from build123d import *

# Parameters (mm, degrees)
F1_DEPTH = 76.2
F2_R     = 4.5085
F3_DEPTH = 92.761762
F4_R     = 6.35
F5_DEPTH = 118.672617


with BuildPart() as f1:
    # F0 (on Front) → F1 (new body)
    with BuildSketch(Plane.XZ):
        Polygon((-46.039158, 105.114406), (-96.838128, 105.437962), (-96.838128, -97.762038), (55.561872, -97.762038), (55.561872, -46.962038), (-46.039158, -46.962038), align=None)
    extrude(amount=F1_DEPTH)

    # F2 (on face) → F3 (cut)
    with BuildSketch(Plane.XY.offset(-46.962038)):
        with Locations((15.037069, -37.766326)):
            Circle(F2_R)
    extrude(amount=-F3_DEPTH, mode=Mode.SUBTRACT)

    # F4 (on face) → F5 (cut)
    with BuildSketch(Plane.YZ.offset(-46.039158)):
        with Locations((-38.88151, 66.329271)):
            Circle(F4_R)
    extrude(amount=-F5_DEPTH, mode=Mode.SUBTRACT)


solid = f1.part
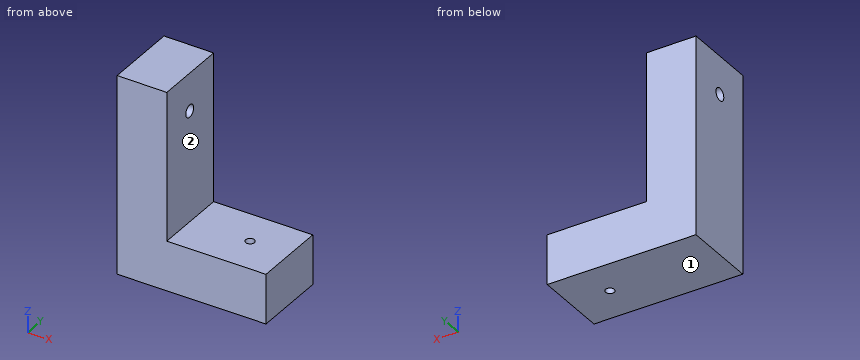
Work out the finished part from the listing and answer in its coordinate system (mm). Face numbers are marked on the shaded views. A direction names the side the tool comes from. Give positions to 0.01 mm unless a question says otherwise; leave off trailing zeros. Order: outer loops, then holes, each group sorted by start corner. A loop starts at its lowest first (then second) coordinate and runs counter-clockwise, first axis right, second up. Notation, with made-up numbers: M 58.5,-25 L 62.5,-25 A22 ccw 62.5,-7 Z; hole C -7,77.5 d10. An arc over 180 degrees is marked long. Return JSON: item names as keys, results as strings.
Q1. Find section B-B, the plane x = -12.5. Write down the section's boundary in (y, z).
Answer below:
{"outline": "M -76.2,-97.76 L 0,-97.76 L 0,-46.96 L -76.2,-46.96 Z"}
Q2. Which of the six approach directions +Z, -Z, +X, -X, +Y, -Y give full straight-line access (tool end or side, diameter ignored) to the marked faces 1 and 2?
Answer below:
{"face 1": "-Z, +X, -X, +Y, -Y", "face 2": "+Z, +X, +Y, -Y"}
Q3. Find section C-C, the plane z = 51. Write down the section's boundary in (x, y).
Answer below:
{"outline": "M -96.84,-76.2 L -46.04,-76.2 L -46.04,0 L -96.84,0 Z"}
Q4. Find section A-A, the plane y = -54. Write down the section's boundary in (x, z), and give its area (3 significant figures).
Answer below:
{"outline": "M -96.84,-97.76 L 55.56,-97.76 L 55.56,-46.96 L -46.04,-46.96 L -46.04,105.11 L -96.84,105.44 Z", "area": "15,500 mm^2"}
Q5. Find the intervals of material crossed by line 1 along Z through (x, y) = (0.5, -42); line 2 along X through (y, z) = (-18, 16); line 3 along Z through (x, y) = (-73, -44), in increasing order. Write a range as [from, to].
Answer below:
{"line 1": "z = [-97.76, -46.96]", "line 2": "x = [-96.84, -46.04]", "line 3": "z = [-97.76, 62.57], [70.09, 105.29]"}
Q6. Each of these flat-tipped pins is pushed along its axis until it touches: pin 1 (6 mm diameter, centred on x = -30.5, y = -38.5, fed in from +Z); pin 2 (1.5 mm diameter, centred on y = -61, z = -28.5, fed in from +X); pin 3 (1.5 mm diameter, centred on x = -57.5, y = -62, fed in from +Z); pin 4 (8 mm diameter, centred on x = 15.04, y = -37.77, fed in from -Z). Where does it stop, or does it pass through?
Answer below:
{"pin 1": "stops at z = -46.96", "pin 2": "stops at x = -46.04", "pin 3": "stops at z = 105.19", "pin 4": "passes through"}
